Verification items for the finished model (mm, model axes). A direction names the side the tool comes from. Give positions to 0.01 mm unless a question says otherwise; leave off trailing zeros. Order: outer loops, then holes, each group sorted by start corner. A loop starts at its lowest first (then second) coordinate and runs counter-clockwise, first axis right, second up.
(1) Gauge pin test, flat ends, axial feed: pin 1 (2 mm diameter, centred on x = 44, y = 8, fed in from +Z); pin 2 (3 mm diameter, centred on y = 1.5, z = 67, fed in from -X); pin 3 (2 mm diameter, centred on x = -59.5, z = -2.5, fed in from -Y). Record the tip position at first contact, or that the pin passes through.
(2) Mould release check, pull along Z, two halves, no side actions. Record for faces 4 (the face through (60, 5, -20)), 5 (the face through (0, 8, 77.5)), 6 (the face through (-19.031, 8.31, 71.863)): pulls with the +Z half, pulls with the -Z half, needs draft (parallel to the pull), parting line crosses it, or undercut.
(3) Sectioned sample at B-B on z = 0.5. Record the cut outline in (x, y), plus the area to 4 significant figures.
(4) Sectioned sample at C-C on y = 9. Count the separate pieces of the cut face and the enclosed holes in it, plus the area to 3 significant figures.
(5) Sectioned sample at D-D on x = 5.5. Record the cut outline in (y, z).
(6) Sectioned sample at A-A on x = -60. Record the cut outline in (y, z).
(7) Access from +Z, -Z, +X, -X, +Y, -Y to the whole of each face (thin tool, end or side, straight path). Record for faces 1 (the face through (-30, 2, 70)), 2 (the face through (-1, 12.5, 17)), 3 (the face through (-70, 2, -20)).
(8) Scan lines: L1, parallel to X at y = 3.25, z = -15.5; L2, parallel to X at y = 1.5, z = -3; L3, parallel to X at y = 5.5, z = -0.5. Record each from-to range of solid material in increasing order.
```python
from build123d import *

# Parameters (mm, degrees)
BOSS_EXTRUDE2_DEPTH = 12.5
SKETCH2_R           = 2.1
BOSS_EXTRUDE3_DEPTH = 29
SKETCH4_W           = 9
SKETCH4_H           = 3.5
CUT_EXTRUDE1_DEPTH  = 73
CHAMFER1_SIZE       = 3
SKETCH5_W           = 60
SKETCH5_H           = 15
SKETCH5_R           = 2.89755201
CUT_EXTRUDE2_DEPTH  = 4
SKETCH6_R           = 2.89755201
CUT_EXTRUDE3_DEPTH  = 26
SKETCH7_R           = 2.1
CUT_EXTRUDE4_DEPTH  = 26
SKETCH8_R           = 2.1
CUT_EXTRUDE5_DEPTH  = 26
SKETCH9_W           = 20
SKETCH9_H           = 45
CUT_EXTRUDE8_DEPTH  = 5
SKETCH10_W          = 1.5
SKETCH10_H          = 3.5
BOSS_EXTRUDE4_DEPTH = 9.75
SKETCH11_R          = 2.1
CUT_EXTRUDE9_DEPTH  = 22
SKETCH12_R          = 2.1
BOSS_EXTRUDE5_DEPTH = 12.5
SKETCH13_W          = 36.022900052
SKETCH13_H          = 69.947378741
CUT_EXTRUDE10_DEPTH = 29
SKETCH14_R          = 2.89755201
SKETCH14_R_2        = 2.1
BOSS_EXTRUDE6_DEPTH = 8.5
SKETCH15_R          = 2.1
CUT_EXTRUDE11_DEPTH = 38
SKETCH16_R          = 2.1
CUT_EXTRUDE12_DEPTH = 38


with BuildPart() as part:
    # Sketch1 → Boss-Extrude2 (new body)
    with BuildSketch(Plane(origin=(0, 0, 0), x_dir=(1, 0, 0), z_dir=(0, 1, 0))):
        Polygon((-80, -42.5), (-80, 42.5), (80, 42.5), (80, -42.5), (30, -77.5), (-30, -77.5), align=None)
    extrude(amount=BOSS_EXTRUDE2_DEPTH)

    # Sketch2 → Boss-Extrude3 (add)
    with BuildSketch(Plane(origin=(0, 12.5, 0), x_dir=(1, 0, 0), z_dir=(0, 1, 0))):
        with BuildLine():
            Line((10.25, -47.5), (-10.25, -47.5))
            Line((-10.25, -47.5), (-10.25, -7))
            Line((-10.25, -7), (-3, -7))
            Line((-3, -7), (-3, -3.640312424))
            ThreePointArc((-3, -3.640312424), (-7.1, -3), (-3, -2.359687576))
            Line((-3, -2.359687576), (-3, 2.75))
            Line((-3, 2.75), (-15, 2.75))
            Line((-15, 2.75), (-15, -57.25))
            Line((-15, -57.25), (15, -57.25))
            Line((15, -57.25), (15, 2.75))
            Line((15, 2.75), (3, 2.75))
            Line((3, 2.75), (3, -2.359687576))
            ThreePointArc((3, -2.359687576), (5.324037035, -0.925150608), (7.1, -3))
            ThreePointArc((7.1, -3), (5.324037035, -5.074849392), (3, -3.640312424))
            Line((3, -3.640312424), (3, -7))
            Line((3, -7), (10.25, -7))
            Line((10.25, -7), (10.25, -47.5))
        make_face()
        with Locations((-5, -51.5)):
            Circle(SKETCH2_R, mode=Mode.SUBTRACT)
        with Locations((5, -51.5)):
            Circle(SKETCH2_R, mode=Mode.SUBTRACT)
    extrude(amount=BOSS_EXTRUDE3_DEPTH)

    # Sketch4 → Cut-Extrude1 (cut)
    with BuildSketch(Plane.XY.offset(57.25)):
        with Locations((5, 35.75)):
            Rectangle(SKETCH4_W, SKETCH4_H)
        with Locations((-5, 35.75)):
            Rectangle(SKETCH4_W, SKETCH4_H)
    extrude(amount=-CUT_EXTRUDE1_DEPTH, mode=Mode.SUBTRACT)

    # Chamfer1
    chamfer1_edges = [part.edges().sort_by_distance(p)[0] for p in [
        (-15, 27, -2.75),
        (-15, 27, 57.25),
        (15, 27, 57.25),
        (15, 27, -2.75),
    ]]
    chamfer(chamfer1_edges, length=CHAMFER1_SIZE)

    # Sketch5 → Cut-Extrude2 (cut)
    with BuildSketch(Plane.XZ):
        with Locations((0, 70)):
            Rectangle(SKETCH5_W, SKETCH5_H)
        with Locations((-20, 70)):
            Circle(SKETCH5_R, mode=Mode.SUBTRACT)
        with Locations((20, 70)):
            Circle(SKETCH5_R, mode=Mode.SUBTRACT)
    extrude(amount=-CUT_EXTRUDE2_DEPTH, mode=Mode.SUBTRACT)

    # Sketch6 → Cut-Extrude3 (cut)
    with BuildSketch(Plane(origin=(0, 0, 0), x_dir=(-1, 0, 0), z_dir=(0, -1, 0))):
        with Locations((20, -70)):
            Circle(SKETCH6_R)
        with Locations((-20, -70)):
            Circle(SKETCH6_R)
    extrude(amount=-CUT_EXTRUDE3_DEPTH, mode=Mode.SUBTRACT)

    # Sketch7 → Cut-Extrude4 (cut)
    with BuildSketch(Plane(origin=(0, 12.5, 0), x_dir=(1, 0, 0), z_dir=(0, 1, 0))):
        with Locations((-75, 32.5)):
            Circle(SKETCH7_R)
        with Locations((-75, 12.5)):
            Circle(SKETCH7_R)
        with Locations((-75, -12.5)):
            Circle(SKETCH7_R)
        with Locations((-75, -32.5)):
            Circle(SKETCH7_R)
        with Locations((75, -32.5)):
            Circle(SKETCH7_R)
        with Locations((75, -12.5)):
            Circle(SKETCH7_R)
        with Locations((75, 12.5)):
            Circle(SKETCH7_R)
        with Locations((75, 32.5)):
            Circle(SKETCH7_R)
    extrude(amount=-CUT_EXTRUDE4_DEPTH, mode=Mode.SUBTRACT)

    # Sketch8 → Cut-Extrude5 (cut)
    with BuildSketch(Plane.XZ):
        with Locations((-60, -6.5)):
            Circle(SKETCH8_R)
        with Locations((-60, -33.5)):
            Circle(SKETCH8_R)
        with Locations((60, -6.5)):
            Circle(SKETCH8_R)
        with Locations((60, -33.5)):
            Circle(SKETCH8_R)
    extrude(amount=-CUT_EXTRUDE5_DEPTH, mode=Mode.SUBTRACT)

    # Sketch9 → Cut-Extrude8 (cut)
    with BuildSketch(Plane.XZ):
        with Locations((-60, -20)):
            Rectangle(SKETCH9_W, SKETCH9_H)
        with Locations((60, -20)):
            Rectangle(SKETCH9_W, SKETCH9_H)
    extrude(amount=-CUT_EXTRUDE8_DEPTH, mode=Mode.SUBTRACT)

    # Sketch10 → Boss-Extrude4 (add)
    with BuildSketch(Plane.XY.offset(57.25)):
        with Locations((0, 35.75)):
            Rectangle(SKETCH10_W, SKETCH10_H)
    extrude(amount=-BOSS_EXTRUDE4_DEPTH)

    # Sketch11 → Cut-Extrude9 (cut)
    with BuildSketch(Plane(origin=(0, 12.5, 0), x_dir=(1, 0, 0), z_dir=(0, 1, 0))):
        with Locations((-42.5, 37.25)):
            Circle(SKETCH11_R)
        with Locations((-42.5, 23.25)):
            Circle(SKETCH11_R)
    extrude(amount=-CUT_EXTRUDE9_DEPTH, mode=Mode.SUBTRACT)

    # Sketch12 → Boss-Extrude5 (add, through all)
    with BuildSketch(Plane(origin=(0, 12.5, 0), x_dir=(1, 0, 0), z_dir=(0, 1, 0))):
        with Locations((-42.5, 37.25)):
            Circle(SKETCH12_R)
        with Locations((-42.5, 23.25)):
            Circle(SKETCH12_R)
    extrude(amount=-BOSS_EXTRUDE5_DEPTH)

    # Sketch13 → Cut-Extrude10 (cut)
    with BuildSketch(Plane(origin=(0, 41.5, 0), x_dir=(1, 0, 0), z_dir=(0, 1, 0))):
        with Locations((0, -27.030330354)):
            Rectangle(SKETCH13_W, SKETCH13_H)
    extrude(amount=-CUT_EXTRUDE10_DEPTH, mode=Mode.SUBTRACT)

    # Sketch14 → Boss-Extrude6 (add)
    with BuildSketch(Plane(origin=(0, 12.5, 0), x_dir=(1, 0, 0), z_dir=(0, 1, 0))):
        with Locations((-20, -70)):
            Circle(SKETCH14_R)
        with Locations((-20, -70)):
            Circle(SKETCH14_R_2, mode=Mode.SUBTRACT)
        with Locations((20, -70)):
            Circle(SKETCH14_R)
        with Locations((20, -70)):
            Circle(SKETCH14_R_2, mode=Mode.SUBTRACT)
    extrude(amount=-BOSS_EXTRUDE6_DEPTH)

    # Sketch15 → Cut-Extrude11 (cut)
    with BuildSketch(Plane(origin=(0, 12.5, 0), x_dir=(1, 0, 0), z_dir=(0, 1, 0))):
        with Locations((-42.53, 15.5)):
            Circle(SKETCH15_R)
        with Locations((-42.53, -0.5)):
            Circle(SKETCH15_R)
        with Locations((42.53, 15.5)):
            Circle(SKETCH15_R)
        with Locations((42.53, -0.5)):
            Circle(SKETCH15_R)
    extrude(amount=-CUT_EXTRUDE11_DEPTH, mode=Mode.SUBTRACT)

    # Sketch16 → Cut-Extrude12 (cut)
    with BuildSketch(Plane(origin=(0, 12.5, 0), x_dir=(1, 0, 0), z_dir=(0, 1, 0))):
        with Locations((35, -47.5)):
            Circle(SKETCH16_R)
        with Locations((35, -67.5)):
            Circle(SKETCH16_R)
        with Locations((60, -47.5)):
            Circle(SKETCH16_R)
    extrude(amount=-CUT_EXTRUDE12_DEPTH, mode=Mode.SUBTRACT)


solid = part.part
```
Ans:
1. pin 1: stops at z = 68.4
1. pin 2: stops at x = -47.14
1. pin 3: stops at y = 5
2. face 4: needs draft
2. face 5: pulls with the +Z half
2. face 6: undercut
3. outline: (-80, 0) - (-70, 0) - (-70, 5) - (-50, 5) - (-50, 0) - (-44.63, 0) - (-44.63, 12.5) - (-80, 12.5) - close; (-40.43, 0) - (40.43, 0) - (40.43, 12.5) - (-40.43, 12.5) - close; (44.63, 0) - (50, 0) - (50, 5) - (70, 5) - (70, 0) - (80, 0) - (80, 12.5) - (44.63, 12.5) - close
3. area: 1,695 mm2
4. separate pieces: 1
4. enclosed holes: 21
4. area: 17,200 mm2
5. outline: (0, -42.5) - (12.5, -42.5) - (12.5, 77.5) - (4, 77.5) - (4, 62.5) - (0, 62.5) - close
6. outline: (0, 2.5) - (5, 2.5) - (5, -4.4) - (12.5, -4.4) - (12.5, 56.5) - (0, 56.5) - close; (5, -42.5) - (12.5, -42.5) - (12.5, -35.6) - (5, -35.6) - close; (5, -31.4) - (12.5, -31.4) - (12.5, -8.6) - (5, -8.6) - close
7. face 1: +Z, -Y
7. face 2: +Z, -Z, +X, -X, +Y
7. face 3: -Z, -Y
8. L1: x = -80 to -70, -50 to -44.63, -40.43 to 40.43, 44.63 to 50, 70 to 80
8. L2: x = -80 to -70, -50 to 50, 70 to 80
8. L3: x = -80 to -44.38, -40.68 to 40.68, 44.38 to 80
